Part model, mm, in its own coordinate system. A direction names the side the tool comes from. Coordinates: 2 decimals unless noted, no trailing zeros. Loops run counter-clockwise (first coordinate to the right, second up) from the corner with the lowest first, then second, coordinate; pieces in that order, holes last. Notation, with made-up numbers: (21.5, -35.5) -> (41.5, -35.5) arc R13 ccw to (41.5, -17.5) -> close; hole circle Ø6 at (60, 77.5). An arc over 180 degrees is marked (long way). Use one line per item in the form item = value. Start each with the question number.
(1) Pin check, flat tips, straight feed: P1, Ø1.6, axis at y = -7.5, z = 5, coming from the +X side; P2, Ø2, axis at x = 0.5, z = 2.5, coming from the -Y side; P3, Ø4, axis at y = 2, z = 3, coming from the -X side. Stop position of each tip, or through.
(2) Band-saw the part on A-A on x = -7.25. Give the cut face in (y, z).
(3) Band-saw the part on C-C on y = -6.25. Give the cut face in (x, z), then the cut area to 3 significant figures.
(4) Band-saw the part on B-B on z = 3.5. Give the cut face in (x, y).
(5) 3-axis set-ups, long thin cutter, end or side, ignore diameter. For faces 4 (the flat face through (-10, -0.25, 3)), 5 (the flat face through (-10.75, -4, 3)), 6 (the flat face through (-3.75, -6, 3)): which of +Z, -Z, +X, -X, +Y, -Y reach the whole face in a straight line?
(6) Mould opens along X. For faces 1 (the cylindrical face through (-7.58, -4.56, 5.98)), 2 (the flat face through (3.75, 0, 3)), 3 (the flat face through (-2.45, 3.25, 3.45)) say: +X half, -X half, draft (parallel to the pull), parting line (faces both ways), or undercut.
(7) Drill centre lines: L1, parallel to Z at x = -7.25, y = -5.75; L2, parallel to X at y = -2.25, z = 1.25; L3, parallel to Z at x = 1.75, y = -2.5. Where is each one in solid material? Low to high. Write a range as [from, to].
(8) Band-saw the part on D-D on x = 0.25. Give the cut face in (y, z), then the cut area to 3 significant figures.
Autodesk Inventor part; units mm, degrees
ref_plane "YZ Plane" through (0, 0, 0) normal (1, 0, 0) x (0, 1, 0)
ref_plane "XZ Plane" through (0, 0, 0) normal (0, 1, 0) x (-1, 0, 0)
ref_plane "XY Plane" through (0, 0, 0) normal (0, 0, 1) x (1, 0, 0)
sketch "スケッチ1" plane through (0, 0, 0) normal (0, 0, 1) x (1, 0, 0)
  line L0 (-3.75, 3.25) -> (3.75, 3.25) construction
  line L1 (3.75, 3.25) -> (3.75, -3.25) construction
  line L2 (3.75, -3.25) -> (-3.75, -3.25) construction
  line L3 (-3.75, -3.25) -> (-3.75, 3.25) construction
  line L4 (0, 0) -> (0, 2.4906) construction
  line L5 (0, 0) -> (2.3218, 0) construction
  line L6 (0.25, 3.25) -> (0.25, -3.25) construction
  line L7 (-2.25, 3.25) -> (-2.25, -3.25) construction
  line L8 (2.75, 3.25) -> (2.75, -3.25) construction
  line L9 (-3.75, 3.25) -> (3.75, -3.25) construction
  line L10 (-3.75, -3.25) -> (3.75, 3.25) construction
  line L11 (-10.75, -0.25) -> (-3.75, -0.25) construction
  line L12 (-3.75, -0.25) -> (-3.75, -8.75) construction
  line L13 (-3.75, -8.75) -> (-10.75, -8.75) construction
  line L14 (-10.75, -8.75) -> (-10.75, -0.25) construction
  line L15 (-10.75, -0.25) -> (-3.75, -8.75) construction
  line L16 (-3.75, -0.25) -> (-10.75, -8.75) construction
  line L17 (-9.75, -0.25) -> (-9.75, -8.75) construction
  line L18 (-4.75, -0.25) -> (-4.75, -8.75) construction
  line L19 (-9.75, -0.25) -> (-4.75, -8.75) construction
  line L20 (-9.75, -8.75) -> (-4.75, -0.25) construction
  line L21 (-7.25, -4.5) -> (-7.25, -8.75) construction
  line L22 (-2.25, 3.25) -> (2.75, -3.25) construction
  line L23 (-2.25, -3.25) -> (2.75, 3.25) construction
  point P0 (-7.25, -4.5)
  dimension "d0" = 5
  dimension "d1" = 6.5
  dimension "d2" = 1
  dimension "d3" = 1.5
  dimension "d31" = 5
  dimension "d32" = 1
  dimension "d33" = 1
  dimension "d34" = 8.5
  dimension "d35" = 3.5
sketch "スケッチ6" plane through (0, 0, 0) normal (0, 0, 1) x (1, 0, 0)
  line L0 (-3.75, 3.25) -> (3.75, 3.25) construction
  line L1 (3.75, 3.25) -> (3.75, -3.25) construction
  line L2 (3.75, -3.25) -> (-3.75, -3.25) construction
  line L3 (-3.75, -3.25) -> (-3.75, 3.25) construction
  line L4 (-2.25, 3.25) -> (-2.25, -3.25) construction
  line L5 (0, 0) -> (0, 2.4906) construction
  line L6 (0, 0) -> (2.3218, 0) construction
  line L7 (0.25, 3.25) -> (0.25, -3.25) construction
  line L8 (-3.75, 3.25) -> (3.75, -3.25) construction
  line L9 (-3.75, -3.25) -> (3.75, 3.25) construction
  line L10 (2.75, 3.25) -> (2.75, -3.25) construction
  line L11 (-3.75, -0.25) -> (-3.75, -8.75) construction
  line L12 (-4.75, -0.25) -> (-4.75, -8.75) construction
  line L13 (-10.75, -0.25) -> (-3.75, -0.25) construction
  line L14 (-9.75, -0.25) -> (-9.75, -8.75) construction
  line L15 (-10.75, -0.25) -> (-3.75, -8.75) construction
  line L16 (-10.75, -8.75) -> (-10.75, -0.25) construction
  line L17 (-3.75, -0.25) -> (-10.75, -8.75) construction
  line L18 (-3.75, -8.75) -> (-10.75, -8.75) construction
  line L19 (-10.75, -0.25) -> (-10.75, -8.75)
  line L20 (-3.75, -8.75) -> (-10.75, -8.75)
  line L21 (-3.75, -8.75) -> (-3.75, -3.25)
  line L22 (-3.75, -3.25) -> (3.75, -3.25)
  line L23 (3.75, -3.25) -> (3.75, 3.25)
  line L24 (3.75, 3.25) -> (-3.75, 3.25)
  line L25 (-3.75, 3.25) -> (-3.75, -0.25)
  line L26 (-10.75, -0.25) -> (-3.75, -0.25)
  line L27 (-2.25, 3.25) -> (2.75, -3.25) construction
  line L28 (-2.25, -3.25) -> (2.75, 3.25) construction
  line L29 (-7.25, -4.5) -> (-7.25, -8.75) construction
  line L30 (-9.75, -0.25) -> (-4.75, -8.75) construction
  line L31 (-9.75, -8.75) -> (-4.75, -0.25) construction
  point P0 (-7.25, -4.5)
extrude "押し出し5" add sketch "スケッチ6" along normal blind 7
ref_plane "作業平面4" through (-10.75, -8.75, 0) normal (0, -1, 0) x (1, 0, 0)
sketch "スケッチ7" plane through (-10.75, -8.75, 0) normal (0, -1, 0) x (1, 0, 0)
  line L0 (7, 7) -> (14.5, 7)
  line L1 (14.5, 7) -> (7, 7)
  line L2 (7, 0) -> (7, 7)
  line L3 (7, 0) -> (14.5, 0)
  line L4 (14.5, 0) -> (14.5, 7)
  line L5 (7, 0) -> (7, 7)
  line L6 (7, 0) -> (7, 7)
  line L7 (14.5, 0) -> (7, 0)
  line L8 (14.5, 0) -> (14.5, 7)
  line L9 (0, 0) -> (0, 7)
  line L10 (0, 0) -> (7, 0)
  line L11 (7, 7) -> (0, 7)
  line L12 (0, 0) -> (0, 7)
  line L13 (7, 0) -> (0, 0)
  line L14 (0, 0) -> (7, 0) construction
  line L15 (1, 0) -> (6, 0) construction
  line L16 (1, 0) -> (6, 0) construction
  line L17 (0, 0) -> (7, 0) construction
  line L18 (7, 0) -> (0, 0) construction
  line L19 (7, 0) -> (0, 0) construction
  line L20 (7, 0) -> (14.5, 0) construction
  line L21 (14.5, 0) -> (7, 0) construction
  line L22 (10.75, 0) -> (13.0718, 0) construction
  line L23 (7, 0) -> (14.5, 0) construction
  line L24 (7, 0) -> (14.5, 0) construction
  line L25 (8.5, 0) -> (13.5, 0) construction
  line L26 (8.5, 0) -> (13.5, 0) construction
  line L27 (3.5, 0) -> (3.5, 7) construction
  line L28 (1, 0) -> (1, 7) construction
  line L29 (6, 0) -> (6, 7) construction
  line L30 (0, 7) -> (7, 7)
  line L31 (1, 7) -> (6, 0) construction
  line L32 (1, 0) -> (6, 7) construction
  circle A0 centre (3.5, 3.5) radius 2.5
  line L33 (8.5, 0) -> (8.5, 7) construction
  line L34 (11, 0) -> (11, 7) construction
  line L35 (13.5, 0) -> (13.5, 7) construction
  line L36 (8.5, 7) -> (13.5, 0) construction
  line L37 (8.5, 0) -> (13.5, 7) construction
  circle A1 centre (11, 3.5) radius 2.5
  point P0 (3.5, 0)
  point P1 (3.5, 0)
  point P2 (10.75, 0)
  point P3 (11, 0)
  dimension "d39" = 5
  dimension "d40" = 5
extrude "押し出し6" cut sketch "スケッチ7" against normal blind 20 contours A0 | A1
properties part number "sensorholder"
A:
q1.P1 = -3.75
q1.P2 = through
q1.P3 = -3.75
q2.outline = (-8.75, 0) -> (-0.25, 0) -> (-0.25, 1) -> (-8.75, 1) -> close; (-8.75, 6) -> (-0.25, 6) -> (-0.25, 7) -> (-8.75, 7) -> close
q3.outline = (-10.75, 0) -> (-3.75, 0) -> (-3.75, 7) -> (-10.75, 7) -> close; hole circle Ø5 at (-7.25, 3.5)
q3.area = 29.4 mm²
q4.outline = (-10.75, -8.75) -> (-9.75, -8.75) -> (-9.75, -0.25) -> (-10.75, -0.25) -> close; (-4.75, -8.75) -> (-3.75, -8.75) -> (-3.75, -3.25) -> (-2.25, -3.25) -> (-2.25, 3.25) -> (-3.75, 3.25) -> (-3.75, -0.25) -> (-4.75, -0.25) -> close; (2.75, -3.25) -> (3.75, -3.25) -> (3.75, 3.25) -> (2.75, 3.25) -> close
q5.face_4 = +Z, -Z, -X, +Y
q5.face_5 = +Z, -Z, -X, +Y, -Y
q5.face_6 = +Z, -Z, +X, -Y
q6.face_1 = undercut
q6.face_2 = +X half
q6.face_3 = draft
q7.L1 = [0, 1], [6, 7]
q7.L2 = [-10.75, -8.34], [-6.16, -0.84], [1.34, 3.75]
q7.L3 = [0, 1.5], [5.5, 7]
q8.outline = (-3.25, 0) -> (3.25, 0) -> (3.25, 1) -> (-3.25, 1) -> close; (-3.25, 6) -> (3.25, 6) -> (3.25, 7) -> (-3.25, 7) -> close
q8.area = 13.0 mm²
